Part print with two shaded views. Sizes in mm from the minimum x, y, z corner. A direction names the side the tool comes from. Give positions to 0.01 mm unless a question says otherwise; leave off trailing zeros. Order: outer loops, then holes, each group sorted by start corner. A loop starts at its lowest first (then second) coordinate and runs counter-clockwise, first axis right, second up. Notation, with made-up numbers: (62, 8) - (82, 8) arc R14 cw to (82, 21) - close; hole circle Ø6 at (13, 83). An arc over 180 degrees is marked (long way). Return JSON: item names as keys, results as strings. Group by question number.
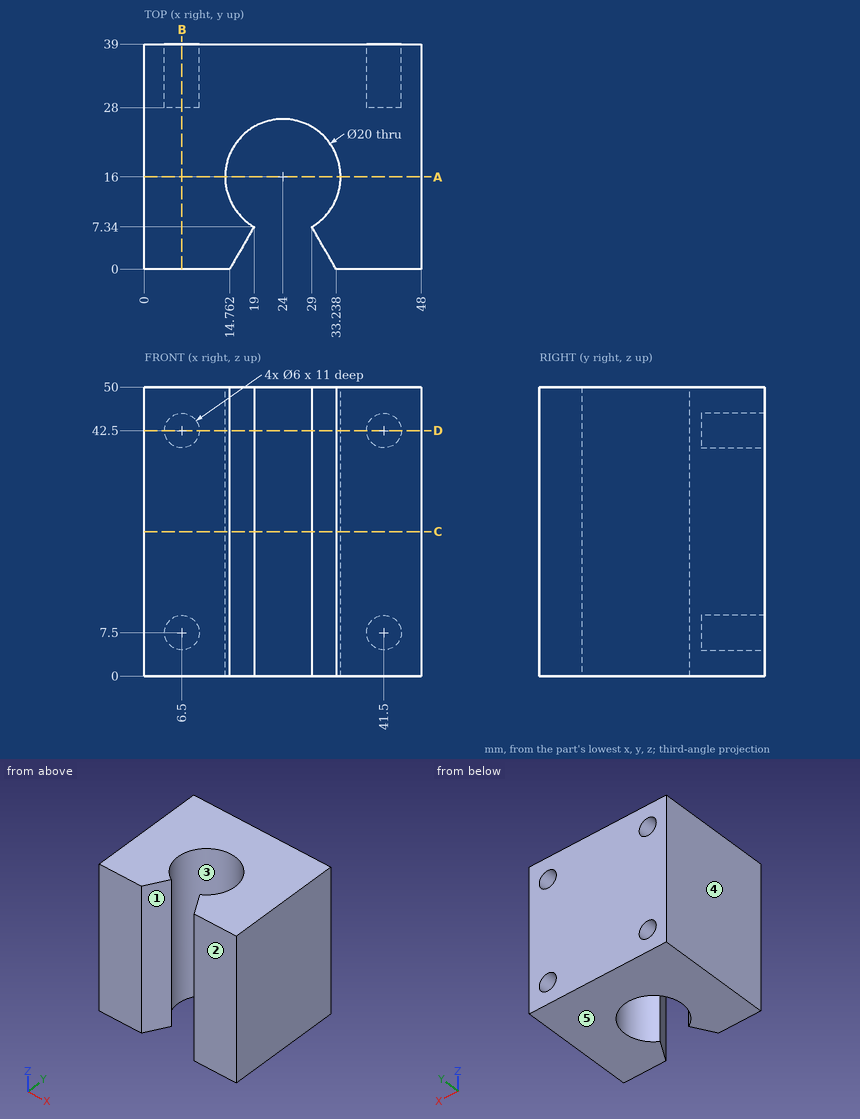
(1) Drop flat-ended pins along their axis: pin 1 Ø1.8 at (x, z) = (41, 8) entering from +Y; pin 2 Ø3 at (x, y) = (34.5, 25) entering from -Z; pin 3 Ø16 at (x, y) = (24, 16) entering from -Z. Give the stop position or say it passes through.
(2) Drill centre lines: L1, parallel to X at y = 32.25, z = 42.5; L2, parallel to X at y = 16, z = 40.5; L3, parallel to X at y = 11.5, z = 22.5. Where is each one in solid material? Low to high.
(3) Slice it at D-D (z = 42.5). Give the cut face in (x, y).
(4) 3-axis set-ups, long thin cutter, end or side, ignore diameter. For the marked faces 1 and 2: which of +Z, -Z, +X, -X, +Y, -Y reach the whole face in a straight line?
(5) Slice it at B-B (x = 6.5). Give the cut face in (y, z), and give its area (3 significant figures).
(6) Pull direction X, two halves, no side cores. Call the marked faces 3, 4 and 5: released by +X, released by -X, zero draft, split by the parting line, or undercut.
(7) Slice it at A-A (y = 16). Give the cut face in (x, z), and give its area (3 significant figures).
(8) Slice it at C-C (z = 25). Give the cut face in (x, y), and give its area (3 significant figures).
Result set:
{
 "1": {"pin 1": "stops at y = 28", "pin 2": "stops at z = 0", "pin 3": "passes through"},
 "2": {"L1": "x = 0 to 3.5, 9.5 to 38.5, 44.5 to 48", "L2": "x = 0 to 14, 34 to 48", "L3": "x = 0 to 15.07, 32.93 to 48"},
 "3": {"outline": "(0, 0) - (14.76, 0) - (19, 7.34) arc R10 cw (long way) to (29, 7.34) - (33.24, 0) - (48, 0) - (48, 39) - (44.5, 39) - (44.5, 28) - (38.5, 28) - (38.5, 39) - (9.5, 39) - (9.5, 28) - (3.5, 28) - (3.5, 39) - (0, 39) - close"},
 "4": {"face 1": "+Z, -Z, -Y", "face 2": "+Z, -Z, +X, -X, -Y"},
 "5": {"outline": "(0, 0) - (39, 0) - (39, 4.5) - (28, 4.5) - (28, 10.5) - (39, 10.5) - (39, 39.5) - (28, 39.5) - (28, 45.5) - (39, 45.5) - (39, 50) - (0, 50) - close", "area": "1,820 mm²"},
 "6": {"face 3": "undercut", "face 4": "released by -X", "face 5": "zero draft"},
 "7": {"outline": "(0, 0) - (14, 0) - (14, 50) - (0, 50) - close; (34, 0) - (48, 0) - (48, 50) - (34, 50) - close", "area": "1,400 mm²"},
 "8": {"outline": "(0, 0) - (14.76, 0) - (19, 7.34) arc R10 cw (long way) to (29, 7.34) - (33.24, 0) - (48, 0) - (48, 39) - (0, 39) - close", "area": "1,460 mm²"}
}
